Here's the drawing with two shaded views (mm, measured from the low corner). I have some questions. A direction names the side the tool comes from. Give positions to 0.01 mm unless a question says otherwise; leave off trailing zeros. Write each loop counter-clockwise with the first axis right and the second up, starting at its lowest first coordinate (ties: lowest second). Pieces come first, ordered by that corner, then holes. Notation, with made-up numbers: (-14, 78.25) -> (5, 78.25) arc R20 cw to (5, 82.25) -> close; hole circle Ø10 at (-24.5, 62.5). An arc over 180 degrees is marked (long way). Put each result on its own line as item: value. Start each with the question number.
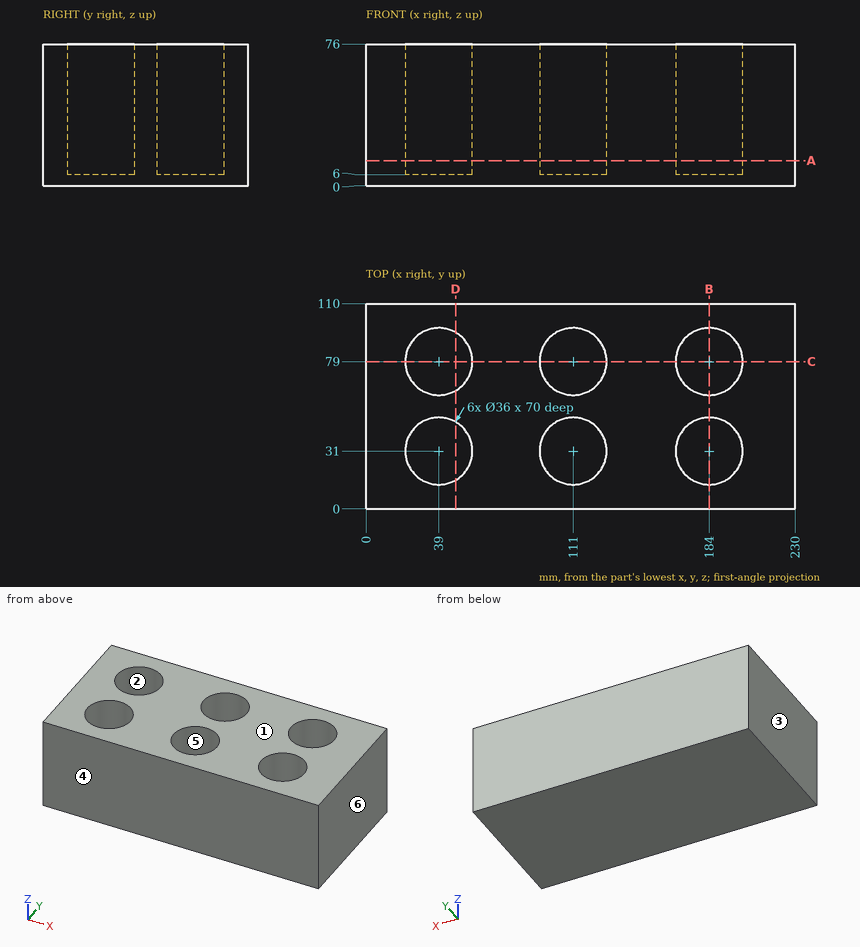
1) I want a section at A-A, the plane z = 13.5. Write out the boundary of the cut face in (x, y).
2) I want a section at C-C, the plane y = 79. Write out the boundary of the cut face in (x, z), and give its area (3 significant figures).
3) I'm going to push a flat-ended pin straight in: pin 1 Ø18 at (x, y) = (43, 85.5) entering from +Z. Where does the tip first touch, or does it pass through?
4) Which directions (+Z, -Z, +X, -X, +Y, -Y) give clear straight access to the entire face, cutting with the end or side of a thin tool? Please do the marked faces 1 and 2.
5) Thinking about a two-plate mould opening in X: for the marked faces 3, 4, 5 and 6, which applies, released by +X, released by -X, zero draft, split by the parting line, or undercut?
6) I want a section at D-D, the plane x = 48. Write out the boundary of the cut face in (y, z).
7) I need wall thicknesses on probe 1 along Y at (x, z) = (184, 57.5); probe 2 along X at (y, z) = (75, 25.5); probe 3 along X at (y, z) = (65.5, 25). Which ranges of each line are inside material? Lowest first, please.
8) I want a section at B-B, the plane x = 184. Write out the boundary of the cut face in (y, z).
Established:
1. outline: (0, 0) -> (230, 0) -> (230, 110) -> (0, 110) -> close; hole circle Ø36 at (39, 31); hole circle Ø36 at (39, 79); hole circle Ø36 at (111, 31); hole circle Ø36 at (111, 79); hole circle Ø36 at (184, 31); hole circle Ø36 at (184, 79)
2. outline: (0, 0) -> (230, 0) -> (230, 76) -> (202, 76) -> (202, 6) -> (166, 6) -> (166, 76) -> (129, 76) -> (129, 6) -> (93, 6) -> (93, 76) -> (57, 76) -> (57, 6) -> (21, 6) -> (21, 76) -> (0, 76) -> close
2. area: 9,920 mm2
3. pin 1: stops at z = 6
4. face 1: +Z, +X, -X, +Y, -Y
4. face 2: +Z
5. face 3: released by -X
5. face 4: zero draft
5. face 5: undercut
5. face 6: released by +X
6. outline: (0, 0) -> (110, 0) -> (110, 76) -> (94.59, 76) -> (94.59, 6) -> (63.41, 6) -> (63.41, 76) -> (46.59, 76) -> (46.59, 6) -> (15.41, 6) -> (15.41, 76) -> (0, 76) -> close
7. probe 1: y = 0 to 13, 49 to 61, 97 to 110
7. probe 2: x = 0 to 21.45, 56.55 to 93.45, 128.55 to 166.45, 201.55 to 230
7. probe 3: x = 0 to 27.09, 50.91 to 99.09, 122.91 to 172.09, 195.91 to 230
8. outline: (0, 0) -> (110, 0) -> (110, 76) -> (97, 76) -> (97, 6) -> (61, 6) -> (61, 76) -> (49, 76) -> (49, 6) -> (13, 6) -> (13, 76) -> (0, 76) -> close
